The listing builds one solid part. Answer for the finished solid, in the listing's coordinates (mm). A direction names the side the tool comes from. Give positions to 0.01 mm unless a question says otherwise; leave off trailing zeros. Loops run counter-clockwise (first coordinate to the right, second up) from the corner with the lowest first, then second, coordinate; pieces in that order, holes last. Notation, with made-up numbers: M 76.5,49.25 L 119.5,49.25 A28 ccw 119.5,67.25 Z; hole C 25.5,79 d4. An arc over 180 degrees is marked long. Use one line per item in the form item = value. Start each with the question number.
1. For faces 4 (the face through (0, -30, 35)), 5 (the face through (-30, 0, 35)), determine the directions among +Z, -Z, +X, -X, +Y, -Y from which every point of the face is accessible in a straight line to the end or side of a thin tool.
2. The part is cut by section A-A (x = 0). Write down the section's boundary in (y, z), and give its area (3 significant figures).
3. The part is cut by section C-C (z = 10). Write down the section's boundary in (x, y), and give its area (3 significant figures).
4. The mould has two halves that part along Y. Classify faces 1 (the face through (0, 35, 35)), 2 (the face through (-25, 0, 35)), 3 (the face through (0, -35, 35)): released by +Y, released by -Y, zero draft, split by the parting line, or undercut.
5. Straight lines are drawn through the part: line 1 (Y direction, x = 0, z = 43.5); line 2 (Z direction, x = 0, y = 31); line 3 (X direction, y = 23, z = 34). For each, find the intervals that lie inside material, in ascending order. Write a range as from..to.
6. The part is cut by section D-D (z = 31). Write down the section's boundary in (x, y), and give its area (3 significant figures).
7. The part is cut by section B-B (x = 9). Write down the section's boundary in (y, z), and give its area (3 significant figures).
from build123d import *

# Parameters (mm, degrees)
F0_W     = 60
F0_H     = 70
F0_W_2   = 50
F0_H_2   = 60
F1_DEPTH = 70
F2_R     = 2
F3_R     = 3.5
F4_DEPTH = 70


with BuildPart() as f1:
    # F0 (on Top) → F1 (new body)
    with BuildSketch(Plane.XY):
        Rectangle(F0_W, F0_H)
        Rectangle(F0_W_2, F0_H_2, mode=Mode.SUBTRACT)
    extrude(amount=F1_DEPTH)

    # F2
    f2_edges = [f1.edges().sort_by_distance(p)[0] for p in [
        (-30, 35, 35),
        (30, 35, 35),
        (30, -35, 35),
        (-30, -35, 35),
        (25, 30, 35),
        (-25, -30, 35),
        (-25, 30, 35),
        (25, -30, 35),
    ]]
    fillet(f2_edges, radius=F2_R)

    # F3 (on face) → F4 (cut)
    with BuildSketch(Plane.XZ.offset(35)):
        with Locations((0, 10)):
            Circle(F3_R)
    extrude(amount=-F4_DEPTH, mode=Mode.SUBTRACT)


solid = f1.part
Derived:
q1.face_4 = +Z, -Z
q1.face_5 = +Z, -Z, -X, +Y, -Y
q2.outline = M -35,0 L -30,0 L -30,6.5 L -35,6.5 Z; M -35,13.5 L -30,13.5 L -30,70 L -35,70 Z; M 30,0 L 35,0 L 35,6.5 L 30,6.5 Z; M 30,13.5 L 35,13.5 L 35,70 L 30,70 Z
q2.area = 630 mm2
q3.outline = M -30,-33 A2 ccw -28,-35 L -3.5,-35 L -3.5,-30 L -23,-30 A2 cw -25,-28 L -25,28 A2 cw -23,30 L -3.5,30 L -3.5,35 L -28,35 A2 ccw -30,33 Z; M 3.5,-35 L 28,-35 A2 ccw 30,-33 L 30,33 A2 ccw 28,35 L 3.5,35 L 3.5,30 L 23,30 A2 cw 25,28 L 25,-28 A2 cw 23,-30 L 3.5,-30 Z
q3.area = 1,130 mm2
q4.face_1 = released by +Y
q4.face_2 = undercut
q4.face_3 = released by -Y
q5.line_1 = -35..-30, 30..35
q5.line_2 = 0..6.5, 13.5..70
q5.line_3 = -30..-25, 25..30
q6.outline = M -30,-33 A2 ccw -28,-35 L 28,-35 A2 ccw 30,-33 L 30,33 A2 ccw 28,35 L -28,35 A2 ccw -30,33 Z; hole M -25,-28 A2 ccw -23,-30 L 23,-30 A2 ccw 25,-28 L 25,28 A2 ccw 23,30 L -23,30 A2 ccw -25,28 Z
q6.area = 1,200 mm2
q7.outline = M -35,0 L -30,0 L -30,70 L -35,70 Z; M 30,0 L 35,0 L 35,70 L 30,70 Z
q7.area = 700 mm2
